from build123d import *

# Parameters (mm, degrees)
EXTRUDE_1_DEPTH     = 20
SKETCH_2_R          = 2.75
CUT_EXTRUDE_1_DEPTH = 36.800621783
SKETCH_3_W          = 5
SKETCH_3_H          = 20
EXTRUDE_2_DEPTH     = 15
SKETCH_4_R          = 2.75
CUT_EXTRUDE_2_DEPTH = 38.697928264
FILLET_1_R          = 2
EXTRUDE_START       = 3
SKETCH_5_R          = 6
SKETCH_5_R_2        = 2.75
EXTRUDE_4_DEPTH     = 3


with BuildPart() as part:
    # 草图1 → 凸台-拉伸1 (new body)
    with BuildSketch(Plane(origin=(0, 0, 0), x_dir=(1, 0, 0), z_dir=(0, 1, 0))):
        Polygon((-12.057971014, 6.222222222), (19.942028986, 6.222222222), (19.942028986, -15.777777778), (14.942028986, -15.777777778), (14.942028986, -10.777777778), (14.942028986, 1.222222222), (-7.057971014, 1.222222222), (-7.057971014, -10.777777778), (-7.057971014, -15.777777778), (-12.057971014, -15.777777778), align=None)
    extrude(amount=EXTRUDE_1_DEPTH)

    # 草图2 → 切除-拉伸1 (cut, through all)
    with BuildSketch(Plane(origin=(0, 0, -6.222222222), x_dir=(-1, 0, 0), z_dir=(0, 0, -1))):
        with Locations((-3.942028986, 10)):
            Circle(SKETCH_2_R)
    extrude(amount=-CUT_EXTRUDE_1_DEPTH, mode=Mode.SUBTRACT)

    # 草图3 → 凸台-拉伸2 (add)
    with BuildSketch(Plane.ZY.offset(12.057971014)):
        with Locations((13.277777778, 10)):
            Rectangle(SKETCH_3_W, SKETCH_3_H)
    extrude_2 = extrude(amount=EXTRUDE_2_DEPTH)

    # 草图4 → 切除-拉伸2 (cut, through all)
    with BuildSketch(Plane(origin=(0, 0, 10.777777778), x_dir=(-1, 0, 0), z_dir=(0, 0, -1))):
        with Locations((19.557971014, 10)):
            Circle(SKETCH_4_R)
    cut_extrude_2 = extrude(amount=-CUT_EXTRUDE_2_DEPTH, mode=Mode.SUBTRACT)

    # 镜向5: 凸台-拉伸2, 切除-拉伸2 across plane
    add(extrude_2.mirror(Plane.ZY.offset(-3.942028986)))
    add(cut_extrude_2.mirror(Plane.ZY.offset(-3.942028986)), mode=Mode.SUBTRACT)

    # 圆角1
    fillet_1_edges = [part.edges().sort_by_distance(p)[0] for p in [
        (-12.057971014, 10, -6.222222222),
        (19.942028986, 10, -6.222222222),
        (-27.057971014, 0, 13.277777778),
        (-27.057971014, 20, 13.277777778),
        (34.942028986, 0, 13.277777778),
        (34.942028986, 20, 13.277777778),
    ]]
    fillet(fillet_1_edges, radius=FILLET_1_R)

    # 草图5 → 凸台-拉伸4 (add)
    with BuildSketch(Plane(origin=(0, 0, -6.222222222), x_dir=(-1, 0, 0), z_dir=(0, 0, -1)).offset(EXTRUDE_START)):
        with Locations(Location((-3.942028986, 10, 0), (0, 0, 180))):
            Circle(SKETCH_5_R)
        with Locations((-3.942028986, 10)):
            Circle(SKETCH_5_R_2, mode=Mode.SUBTRACT)
    extrude(amount=-EXTRUDE_4_DEPTH)


solid = part.part
Geometry check sheet. Reference: the model listing, model coordinates, mm. A direction names the side the tool comes from. Coordinates: 2 decimals unless noted, no trailing zeros. Write each loop counter-clockwise with the first axis right and the second up, starting at its lowest first coordinate (ties: lowest second). Pieces come first, ordered by that corner, then holes. Notation, with made-up numbers: (67.5, -33) -> (106.5, -33) arc R22 ccw to (106.5, -2) -> close; hole circle Ø6 at (10.5, 88.25). An arc over 180 degrees is marked (long way). One line per question, with ' | ' between items.
1. Cross-section at D-D on y = 2.75. Record the cut outline in (x, z).
Answers:
outline: (-27.06, 10.78) -> (-12.06, 10.78) -> (-12.06, -4.22) arc R2 ccw to (-10.06, -6.22) -> (17.94, -6.22) arc R2 ccw to (19.94, -4.22) -> (19.94, 10.78) -> (34.94, 10.78) -> (34.94, 15.78) -> (14.94, 15.78) -> (14.94, -1.22) -> (-7.06, -1.22) -> (-7.06, 15.78) -> (-27.06, 15.78) -> close
2. Draft check along Y on faces 1 (the cylindrical face through (19.37, 10.14, -5.62)), 2 (the cylindrical face through (27.084, 12.727, 13.243)), 3 (the cylindrical face through (3.16, 4.05, -7.74)). Enter one of: +Y half, -Y half, draft (parallel to the pull), parting line (faces both ways), or undercut.
Answers:
face 1: draft | face 2: undercut | face 3: parting line
3. Set-up check for faces 4 (the flat face through (-12.058, 10, 3)), 5 (the cylindrical face through (-22.18, 10.83, 13.24)), 6 (the flat face through (-7.058, 10, 7)), 7 (the flat face through (25.7, 7.6, 10.778)): record each of +Z, -Z, +X, -X, +Y, -Y from which the full face is reachable in a straight line by a thin tool's end or side.
Answers:
face 4: -Z, -X, +Y, -Y | face 5: +Z, -Z | face 6: +Z, +Y, -Y | face 7: -Z, +X, +Y, -Y
4. Cross-section at A-A on z = 13. Record the cut outline in (x, y).
Answers:
outline: (-27.06, 2) arc R2 ccw to (-25.06, 0) -> (-7.06, 0) -> (-7.06, 20) -> (-25.06, 20) arc R2 ccw to (-27.06, 18) -> close; (14.94, 0) -> (32.94, 0) arc R2 ccw to (34.94, 2) -> (34.94, 18) arc R2 ccw to (32.94, 20) -> (14.94, 20) -> close; hole circle Ø5.5 at (-19.56, 10); hole circle Ø5.5 at (27.44, 10)
5. Depth check by flat-ended pin: pin 1 Ø12 at (x, y) = (24, 11) entering from -Z; pin 2 Ø2 at (y, z) = (15.5, -2.5) entering from -X; pin 3 Ø5 at (x, y) = (27.44, 10) entering from -Z; pin 4 Ø4.5 at (y, z) = (9, 1.5) entering from +X. Enter the tip coordinate at first touch or a pass-through.
Answers:
pin 1: stops at z = -6.22 | pin 2: stops at x = -12.06 | pin 3: passes through | pin 4: stops at x = 19.94
6. Cross-section at B-B on y = 10. State how many separate pieces and enclosed holes the cut face has, and give its area (3 significant figures).
Answers:
separate pieces: 4 | enclosed holes: 0 | area: 415 mm²
7. Thickness scan on probe 1 along X at (y, z) = (17.75, 0.5); probe 2 along X at (y, z) = (2, 14.75); probe 3 along Z at (x, y) = (6, 16.25). Record the ranges inside material, lowest first. Write a range as from..to.
Answers:
probe 1: x = -12.06..-7.06, 14.94..19.94 | probe 2: x = -27.06..-7.06, 14.94..34.94 | probe 3: z = -6.22..-1.22
8. Cross-section at C-C on x = 6. Record the cut outline in (y, z), and give its area (3 significant figures).
Answers:
outline: (0, -6.22) -> (4.36, -6.22) -> (4.36, -9.22) -> (8.18, -9.22) -> (8.18, -1.22) -> (0, -1.22) -> close; (11.82, -9.22) -> (15.64, -9.22) -> (15.64, -6.22) -> (20, -6.22) -> (20, -1.22) -> (11.82, -1.22) -> close | area: 105 mm²
